from build123d import *

# Parameters (mm, degrees)
BOSS_EXTRUDE1_DEPTH = 10
FILLET1_R           = 20
BOSS_EXTRUDE2_START = 180
BOSS_EXTRUDE2_DEPTH = 180
BOSS_EXTRUDE3_START = 15
BOSS_EXTRUDE3_DEPTH = 15
BOSS_EXTRUDE4_DEPTH = 15
BOSS_EXTRUDE5_START = 15
SKETCH4_3_R         = 11
BOSS_EXTRUDE5_DEPTH = 38


with BuildPart() as part:
    # Sketch1 → Boss-Extrude1 (new body)
    with BuildSketch(Plane.XY):
        Polygon((-335.812036678, 398.75165032), (309.187963322, 398.75165032), (309.187963322, 68.75165032), (116.024594022, 68.75165032), (116.024594022, -251.24834968), (309.187963322, -251.24834968), (309.187963322, -581.24834968), (-335.812036678, -581.24834968), (-335.812036678, -206.24834968), (-455.812036678, -206.24834968), (-455.812036678, 23.75165032), (-335.812036678, 23.75165032), align=None)
    extrude(amount=BOSS_EXTRUDE1_DEPTH)

    # Fillet1
    fillet1_edges = [part.edges().sort_by_distance(p)[0] for p in [
        (-335.812036678, -206.24834968, 5),
        (-455.812036678, -206.24834968, 5),
        (-455.812036678, 23.75165032, 5),
        (-335.812036678, 23.75165032, 5),
        (-335.812036678, 398.75165032, 5),
        (309.187963322, 398.75165032, 5),
        (309.187963322, 68.75165032, 5),
        (116.024594022, 68.75165032, 5),
        (116.024594022, -251.24834968, 5),
        (309.187963322, -251.24834968, 5),
        (309.187963322, -581.24834968, 5),
        (-335.812036678, -581.24834968, 5),
    ]]
    fillet(fillet1_edges, radius=FILLET1_R)

    # Sketch2 → Boss-Extrude2 (add)
    with BuildSketch(Plane.XY.offset(10).offset(BOSS_EXTRUDE2_START)):
        with BuildLine():
            Line((309.187963322, 88.75165032), (309.187963322, 378.75165032))
            ThreePointArc((309.187963322, 378.75165032), (303.330098945, 392.893785944), (289.187963322, 398.75165032))
            Line((289.187963322, 398.75165032), (-315.812036678, 398.75165032))
            ThreePointArc((-315.812036678, 398.75165032), (-329.954172302, 392.893785944), (-335.812036678, 378.75165032))
            Line((-335.812036678, 378.75165032), (-335.812036678, 43.75165032))
            ThreePointArc((-335.812036678, 43.75165032), (-341.669901055, 29.609514696), (-355.812036678, 23.75165032))
            Line((-355.812036678, 23.75165032), (-435.812036678, 23.75165032))
            ThreePointArc((-435.812036678, 23.75165032), (-449.954172302, 17.893785944), (-455.812036678, 3.75165032))
            Line((-455.812036678, 3.75165032), (-455.812036678, -186.24834968))
            ThreePointArc((-455.812036678, -186.24834968), (-449.954172302, -200.390485304), (-435.812036678, -206.24834968))
            Line((-435.812036678, -206.24834968), (-355.812036678, -206.24834968))
            ThreePointArc((-355.812036678, -206.24834968), (-341.669901055, -212.106214056), (-335.812036678, -226.24834968))
            Line((-335.812036678, -226.24834968), (-335.812036678, -561.24834968))
            ThreePointArc((-335.812036678, -561.24834968), (-329.954172302, -575.390485304), (-315.812036678, -581.24834968))
            Line((-315.812036678, -581.24834968), (289.187963322, -581.24834968))
            ThreePointArc((289.187963322, -581.24834968), (303.330098945, -575.390485304), (309.187963322, -561.24834968))
            Line((309.187963322, -561.24834968), (309.187963322, -271.24834968))
            ThreePointArc((309.187963322, -271.24834968), (303.330098945, -257.106214056), (289.187963322, -251.24834968))
            Line((289.187963322, -251.24834968), (136.024594022, -251.24834968))
            ThreePointArc((136.024594022, -251.24834968), (121.882458398, -245.390485304), (116.024594022, -231.24834968))
            Line((116.024594022, -231.24834968), (116.024594022, 48.75165032))
            ThreePointArc((116.024594022, 48.75165032), (121.882458398, 62.893785944), (136.024594022, 68.75165032))
            Line((136.024594022, 68.75165032), (289.187963322, 68.75165032))
            ThreePointArc((289.187963322, 68.75165032), (303.330098945, 74.609514696), (309.187963322, 88.75165032))
        make_face()
        with BuildLine():
            Line((299.187963322, 88.75165032), (299.187963322, 378.75165032))
            ThreePointArc((299.187963322, 378.75165032), (296.259031134, 385.822718132), (289.187963322, 388.75165032))
            Line((289.187963322, 388.75165032), (-315.812036678, 388.75165032))
            ThreePointArc((-315.812036678, 388.75165032), (-322.88310449, 385.822718132), (-325.812036678, 378.75165032))
            Line((-325.812036678, 378.75165032), (-325.812036678, 43.75165032))
            ThreePointArc((-325.812036678, 43.75165032), (-334.598833243, 22.538446884), (-355.812036678, 13.75165032))
            Line((-355.812036678, 13.75165032), (-435.812036678, 13.75165032))
            ThreePointArc((-435.812036678, 13.75165032), (-442.88310449, 10.822718132), (-445.812036678, 3.75165032))
            Line((-445.812036678, 3.75165032), (-445.812036678, -186.24834968))
            ThreePointArc((-445.812036678, -186.24834968), (-442.88310449, -193.319417492), (-435.812036678, -196.24834968))
            Line((-435.812036678, -196.24834968), (-355.812036678, -196.24834968))
            ThreePointArc((-355.812036678, -196.24834968), (-334.598833243, -205.035146245), (-325.812036678, -226.24834968))
            Line((-325.812036678, -226.24834968), (-325.812036678, -561.24834968))
            ThreePointArc((-325.812036678, -561.24834968), (-322.88310449, -568.319417492), (-315.812036678, -571.24834968))
            Line((-315.812036678, -571.24834968), (289.187963322, -571.24834968))
            ThreePointArc((289.187963322, -571.24834968), (296.259031134, -568.319417492), (299.187963322, -561.24834968))
            Line((299.187963322, -561.24834968), (299.187963322, -271.24834968))
            ThreePointArc((299.187963322, -271.24834968), (296.259031134, -264.177281868), (289.187963322, -261.24834968))
            Line((289.187963322, -261.24834968), (136.024594022, -261.24834968))
            ThreePointArc((136.024594022, -261.24834968), (114.811390587, -252.461553116), (106.024594022, -231.24834968))
            Line((106.024594022, -231.24834968), (106.024594022, 48.75165032))
            ThreePointArc((106.024594022, 48.75165032), (114.811390587, 69.964853755), (136.024594022, 78.75165032))
            Line((136.024594022, 78.75165032), (289.187963322, 78.75165032))
            ThreePointArc((289.187963322, 78.75165032), (296.259031134, 81.680582508), (299.187963322, 88.75165032))
        make_face(mode=Mode.SUBTRACT)
    extrude(amount=-BOSS_EXTRUDE2_DEPTH)

    # Sketch3 → Boss-Extrude3 (add)
    with BuildSketch(Plane.XY.offset(190).offset(BOSS_EXTRUDE3_START)):
        with BuildLine():
            Line((309.187963322, 88.75165032), (309.187963322, 378.75165032))
            ThreePointArc((309.187963322, 378.75165032), (303.330098945, 392.893785944), (289.187963322, 398.75165032))
            Line((289.187963322, 398.75165032), (-315.812036678, 398.75165032))
            ThreePointArc((-315.812036678, 398.75165032), (-329.954172302, 392.893785944), (-335.812036678, 378.75165032))
            Line((-335.812036678, 378.75165032), (-335.812036678, 43.75165032))
            ThreePointArc((-335.812036678, 43.75165032), (-341.669901055, 29.609514696), (-355.812036678, 23.75165032))
            Line((-355.812036678, 23.75165032), (-435.812036678, 23.75165032))
            ThreePointArc((-435.812036678, 23.75165032), (-449.954172302, 17.893785944), (-455.812036678, 3.75165032))
            Line((-455.812036678, 3.75165032), (-455.812036678, -186.24834968))
            ThreePointArc((-455.812036678, -186.24834968), (-449.954172302, -200.390485304), (-435.812036678, -206.24834968))
            Line((-435.812036678, -206.24834968), (-355.812036678, -206.24834968))
            ThreePointArc((-355.812036678, -206.24834968), (-341.669901055, -212.106214056), (-335.812036678, -226.24834968))
            Line((-335.812036678, -226.24834968), (-335.812036678, -561.24834968))
            ThreePointArc((-335.812036678, -561.24834968), (-329.954172302, -575.390485304), (-315.812036678, -581.24834968))
            Line((-315.812036678, -581.24834968), (289.187963322, -581.24834968))
            ThreePointArc((289.187963322, -581.24834968), (303.330098945, -575.390485304), (309.187963322, -561.24834968))
            Line((309.187963322, -561.24834968), (309.187963322, -271.24834968))
            ThreePointArc((309.187963322, -271.24834968), (303.330098945, -257.106214056), (289.187963322, -251.24834968))
            Line((289.187963322, -251.24834968), (136.024594022, -251.24834968))
            ThreePointArc((136.024594022, -251.24834968), (121.882458398, -245.390485304), (116.024594022, -231.24834968))
            Line((116.024594022, -231.24834968), (116.024594022, 48.75165032))
            ThreePointArc((116.024594022, 48.75165032), (121.882458398, 62.893785944), (136.024594022, 68.75165032))
            Line((136.024594022, 68.75165032), (289.187963322, 68.75165032))
            ThreePointArc((289.187963322, 68.75165032), (303.330098945, 74.609514696), (309.187963322, 88.75165032))
        make_face()
    extrude(amount=-BOSS_EXTRUDE3_DEPTH)

    # Sketch4 → Boss-Extrude4 (add)
    with BuildSketch(Plane.ZY.offset(455.812036678)):
        with BuildLine():
            Line((60, -32.244741311), (60, -158.524628982))
            ThreePointArc((60, -158.524628982), (40, -178.524628982), (20, -158.524628982))
            Line((20, -158.524628982), (20, -32.244741311))
            ThreePointArc((20, -32.244741311), (40, -12.244741311), (60, -32.244741311))
        make_face()
    extrude(amount=BOSS_EXTRUDE4_DEPTH)

    # Sketch4<3> → Boss-Extrude5 (add)
    with BuildSketch(Plane.ZY.offset(455.812036678).offset(BOSS_EXTRUDE5_START)):
        with Locations(Location((40, -144.762351153, 0), (0, 0, 270))):
            Circle(SKETCH4_3_R)
        with Locations(Location((40, -118.868830691, 0), (0, 0, 270))):
            Circle(SKETCH4_3_R)
        with Locations(Location((40, -87.715688885, 0), (0, 0, 270))):
            Circle(SKETCH4_3_R)
        with Locations(Location((40, -60.203823394, 0), (0, 0, 270))):
            Circle(SKETCH4_3_R)
        with Locations(Location((40, -33.09654416, 0), (0, 0, 270))):
            Circle(SKETCH4_3_R)
    extrude(amount=BOSS_EXTRUDE5_DEPTH)


solid = part.part
Verification items for the finished model (mm, model axes). A direction names the side the tool comes from. Give positions to 0.01 mm unless a question says otherwise; leave off trailing zeros. Loops run counter-clockwise (first coordinate to the right, second up) from the corner with the lowest first, then second, coordinate; pieces in that order, holes last.
1) Thickness scan on line 1 along Y through (x, z) = (-422.5, 42); line 2 along Y through (x, z) = (29, 41); line 3 along X through (y, z) = (122, 82.5). Record the ranges inside material, lowest first.
2) Sectioned sample at A-A, the plane x = -180.5. Enter the section's corners in (y, z), then the cut area to 3 significant figures.
3) Sectioned sample at B-B, the plane y = 189. Enter the section's corners in (x, z), then the cut area to 3 significant figures.
4) Depth check by flat-ended pin: pin 1 Ø4 at (x, y) = (-20.5, -59.5) entering from -Z; pin 2 Ø16.5 at (x, y) = (-465, -91) entering from -Z; pin 3 Ø1 at (y, z) = (-91, 107.5) entering from -X; pin 4 Ø4 at (y, z) = (128.5, 111.5) entering from -X. Enter the tip coordinate at first touch or a pass-through.
5) Set-up check for faces 1 (the cylindrical face through (-489.546, -39.01, 49.275)), 2 (the cylindrical face through (-463.21, -178.52, 40.44)), 3 (the flat face through (212, 68.752, 104)): record each of +Z, -Z, +X, -X, +Y, -Y from which the full face is reachable in a straight line by a thin tool's end or side.
6) Draft check along X on faces 4 (the flat face through (-79, -85, 190)), 5 (the flat face through (-18, -581.248, 104)), 6 (the cylindrical face through (303.48, -257.26, 103.94)). Enter one of: pulls with the +X half, pulls with the -X half, needs draft (parallel to the pull), parting line crosses it, or undercut.
Answers:
1. line 1: y = -206.25 to -196.25, 13.75 to 23.75
1. line 2: y = -581.25 to -571.25, 388.75 to 398.75
1. line 3: x = -335.81 to -325.81, 299.19 to 309.19
2. outline: (-581.25, 0) - (398.75, 0) - (398.75, 205) - (-581.25, 205) - close; hole (-571.25, 10) - (388.75, 10) - (388.75, 190) - (-571.25, 190) - close
2. area: 28,100 mm2
3. outline: (-335.81, 0) - (309.19, 0) - (309.19, 205) - (-335.81, 205) - close; hole (-325.81, 10) - (299.19, 10) - (299.19, 190) - (-325.81, 190) - close
3. area: 19,700 mm2
4. pin 1: stops at z = 0
4. pin 2: stops at z = 20
4. pin 3: stops at x = -455.81
4. pin 4: stops at x = -335.81
5. face 1: -X
5. face 2: -X, -Y
5. face 3: +Z, -Z, +X
6. face 4: undercut
6. face 5: needs draft
6. face 6: pulls with the +X half
